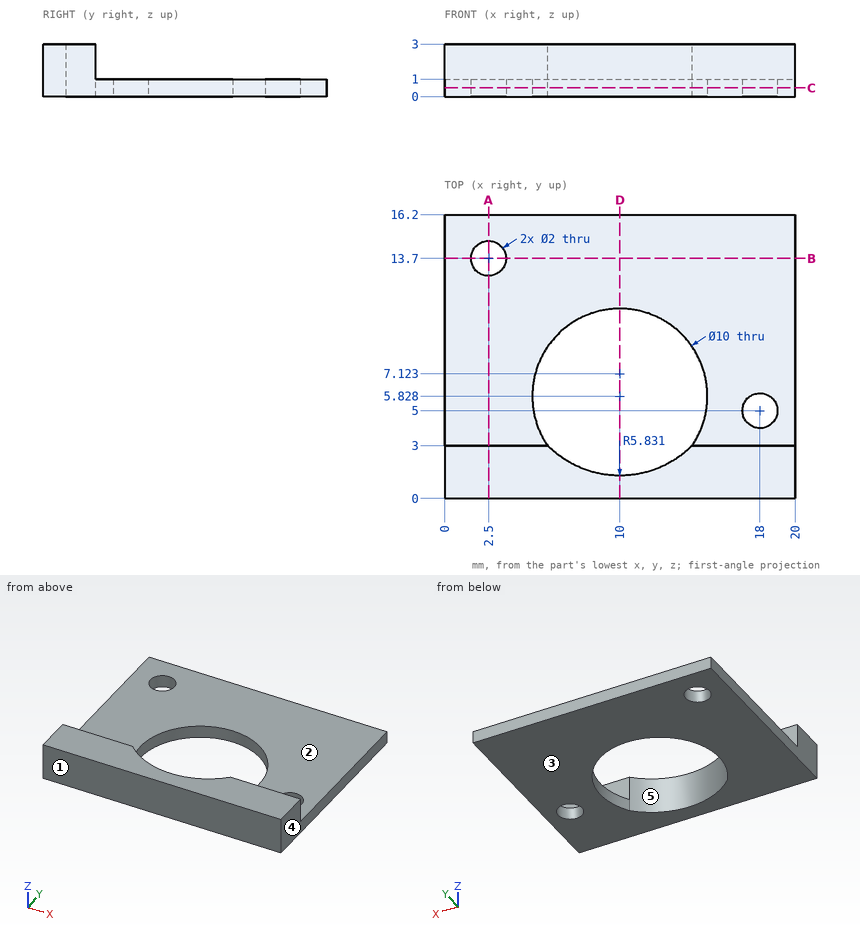
Answer from the drawing. Dimensions are ordinates in mm from the lowest x, y and z of the part. A direction names the side the tool comes from. Give positions to 0.01 mm unless a question says otherwise; leave off trailing zeros. Order: outer loops, then holes, each group sorted by start corner. A loop starts at its lowest first (then second) coordinate and runs counter-clockwise, first axis right, second up.
(1) Find section B-B (y = 13.7). Give the vertices of the cut face in (x, z).
(2) Find section D-D (x = 10). Give the vertices of the cut face in (y, z).
(3) Find section A-A (x = 2.5). Give the vertices of the cut face in (y, z).
(4) For the marked faces 1 and 2, determine the directions among +Z, -Z, +X, -X, +Y, -Y from which every point of the face is accessible in a straight line to the end or side of a thin tool.
(5) Straight lines are drawn through the part: L1, parallel to Y at x = 18, z = 0.7; L2, parallel to Y at x = 2.5, z = 0.7; L3, parallel to Z at x = 13.5, y = 13.5. For each, find the intervals that lie inside material, in ascending order.
(6) Given pin 1 (1.5 mm diameter, centred on x = 15.5, y = 6, fed in from -Z); pin 2 (0.6 mm diameter, centred on x = 18, z = 2.5, fed in from +Y); pin 3 (1.5 mm diameter, centred on x = 7.5, z = 2.5, fed in from +Y), each flat-ended and moving along its own axis, determine where each tip first touches the part or whether it passes through.
(7) Find section C-C (z = 0.5). Give the vertices of the cut face in (x, y).
(8) For a pull along X with two mould halves and no side action, classify the marked faces 3, 4 and 5 as released by +X, released by -X, zero draft, split by the parting line, or undercut.
Result sheet:
1. outline: (0, 0) - (1.5, 0) - (1.5, 1) - (0, 1) - close; (3.5, 0) - (20, 0) - (20, 1) - (3.5, 1) - close
2. outline: (0, 0) - (1.29, 0) - (1.29, 3) - (0, 3) - close; (10.83, 0) - (16.2, 0) - (16.2, 1) - (10.83, 1) - close
3. outline: (0, 0) - (12.7, 0) - (12.7, 1) - (3, 1) - (3, 3) - (0, 3) - close; (14.7, 0) - (16.2, 0) - (16.2, 1) - (14.7, 1) - close
4. face 1: +Z, -Z, +X, -X, -Y
4. face 2: +Z, +X, -X, +Y
5. L1: y = 0 to 4, 6 to 16.2
5. L2: y = 0 to 12.7, 14.7 to 16.2
5. L3: z = 0 to 1
6. pin 1: stops at z = 0
6. pin 2: stops at y = 3
6. pin 3: stops at y = 2.28
7. outline: (0, 0) - (20, 0) - (20, 16.2) - (0, 16.2) - close; hole circle Ø2 at (2.5, 13.7); hole (5.88, 3) arc R5.83 ccw to (14.12, 3) arc R5 ccw (long way) to start; hole circle Ø2 at (18, 5)
8. face 3: zero draft
8. face 4: released by +X
8. face 5: undercut
